Input: part model. Units: mm. Frame: model coordinates. A direction names the side the tool comes from. Round coordinates to 2 decimals unless told otherwise and drop trailing zeros. Loops run counter-clockwise (first coordinate to the right, second up) from the corner with the lowest first, then second, coordinate; pieces in that order, holes last. Notation, with made-up numbers: (71, 38.5) -> (128, 38.5) arc R31 cw to (128, 68.5) -> close; hole circle Ø4 at (56.25, -23). An arc over 180 degrees is marked (long way). Answer as a JSON object with one key per item and string values. Group by question number.
Item 1: Set-up query: faces 1 (the flat face through (9, 48, -20)), 2 (the flat face through (9, -46, -10)), 3 (the flat face through (9, -42, -5)). Return all of +Z, -Z, +X, -X, +Y, -Y with unobstructed straight access to the full face (end or side cutting, diameter ignored); none if empty.
Item 2: Material intervals for line 1 (Y direction, x = 1.1, z = -7.5); line 2 (X direction, y = 57, z = 2); line 3 (Y direction, x = 11.5, z = -4), sorted ascending. Write a range as [from, to].
Item 3: Draft query along Y for faces 4 (the cylindrical face through (8.87, 0.92, 41.99)), 5 (the flat face through (9, 50, -10)), 6 (the cylindrical face through (0.986, 57.737, -7.695)), 7 (the flat face through (0, 27, 33)). Return one class per face: released by +Y, released by -Y, zero draft, split by the parting line, or undercut.
Item 4: Pin query (flat end, axial travel): pin 1 (5.5 mm diameter, centred on x = 10.5, z = -13, fed in from -Y); pin 2 (8 mm diameter, centred on x = 3.5, y = -3, fed in from +Z); pin 3 (6 mm diameter, centred on y = 38, z = 23, fed in from -X); pin 4 (1.5 mm diameter, centred on x = 12, y = 29.5, fed in from -Z). Return the tip coordinate at first contact, or that it passes through.
Item 5: Section query D-D on y = 0. Return loops of the section in (x, z), and give its area (3 significant figures).
Item 6: Section query B-B on z = 20.5. Return loops of the section in (x, y), and give its area (3 significant figures).
Item 7: Section query A-A on z = -7.5. Return loops of the section in (x, y), and give its area (3 significant figures).
Item 8: Section query C-C on x = 4.75. Return loops of the section in (y, z).
from build123d import *

# Parameters (mm, degrees)
BOSS_EXTRUDE1_DEPTH = 18
SKETCH2_W           = 25
SKETCH2_H           = 16.5
BOSS_EXTRUDE2_DEPTH = 2
SKETCH3_W           = 25
SKETCH3_H           = 16.5
BOSS_EXTRUDE3_DEPTH = 2
SKETCH4_R           = 1.5
CUT_EXTRUDE1_DEPTH  = 32
FILLET1_R           = 10


with BuildPart() as part:
    # Sketch1 → Boss-Extrude1 (new body)
    with BuildSketch(Plane(origin=(0, 0, 0), x_dir=(0, 0, -1), z_dir=(1, 0, 0))):
        with BuildLine():
            Line((0, -42), (10, -42))
            Line((10, -42), (10, -50))
            Line((10, -50), (0, -50))
            ThreePointArc((0, -50), (-50, 0), (0, 50))
            Line((0, 50), (20, 50))
            Line((20, 50), (20, 42))
            Line((20, 42), (0, 42))
            ThreePointArc((0, 42), (-42, 0), (0, -42))
        make_face()
    extrude(amount=BOSS_EXTRUDE1_DEPTH)

    # Sketch2 → Boss-Extrude2 (add)
    with BuildSketch(Plane(origin=(18, 0, 0), x_dir=(0, 0, -1), z_dir=(1, 0, 0))):
        with Locations((7.5, 54.25)):
            Rectangle(SKETCH2_W, SKETCH2_H)
    extrude(amount=-BOSS_EXTRUDE2_DEPTH)

    # Sketch3 → Boss-Extrude3 (add)
    with BuildSketch(Plane.ZY):
        with Locations((-7.5, 54.25)):
            Rectangle(SKETCH3_W, SKETCH3_H)
    extrude(amount=-BOSS_EXTRUDE3_DEPTH)

    # Sketch4 → Cut-Extrude1 (cut)
    with BuildSketch(Plane.ZY):
        with Locations((-7.5, 56.25)):
            Circle(SKETCH4_R)
    extrude(amount=-CUT_EXTRUDE1_DEPTH, mode=Mode.SUBTRACT)

    # Fillet1
    fillet1_edges = [part.edges().sort_by_distance(p)[0] for p in [
        (17, 62.5, 5),
        (1, 62.5, 5),
    ]]
    fillet(fillet1_edges, radius=FILLET1_R)


solid = part.part
Solved:
{
 "1": {"face 1": "-Z, +X, -X, +Y, -Y", "face 2": "-Z, +X, -X, -Y", "face 3": "-Z, +X, -X"},
 "2": {"line 1": "[-50, -42], [42, 54.75], [57.75, 62.5]", "line 2": "[0, 2], [16, 18]", "line 3": "[-50, -42], [42, 50]"},
 "3": {"face 4": "undercut", "face 5": "released by +Y", "face 6": "undercut", "face 7": "zero draft"},
 "4": {"pin 1": "y = 42", "pin 2": "z = 50", "pin 3": "x = 0", "pin 4": "z = 29.14"},
 "5": {"outline": "(0, 42) -> (18, 42) -> (18, 50) -> (0, 50) -> close", "area": "144 mm²"},
 "6": {"outline": "(0, -45.6) -> (18, -45.6) -> (18, -36.66) -> (0, -36.66) -> close; (0, 36.66) -> (18, 36.66) -> (18, 45.6) -> (0, 45.6) -> close", "area": "322 mm²"},
 "7": {"outline": "(0, -50) -> (18, -50) -> (18, -42) -> (0, -42) -> close; (0, 42) -> (18, 42) -> (18, 54.75) -> (16, 54.75) -> (16, 50) -> (2, 50) -> (2, 54.75) -> (0, 54.75) -> close; (0, 57.75) -> (2, 57.75) -> (2, 62.5) -> (0, 62.5) -> close; (16, 57.75) -> (18, 57.75) -> (18, 62.5) -> (16, 62.5) -> close", "area": "326 mm²"},
 "8": {"outline": "(-50, -10) -> (-42, -10) -> (-42, 0) arc R42 cw to (42, 0) -> (42, -20) -> (50, -20) -> (50, 0) arc R50 ccw to (-50, 0) -> close"}
}
